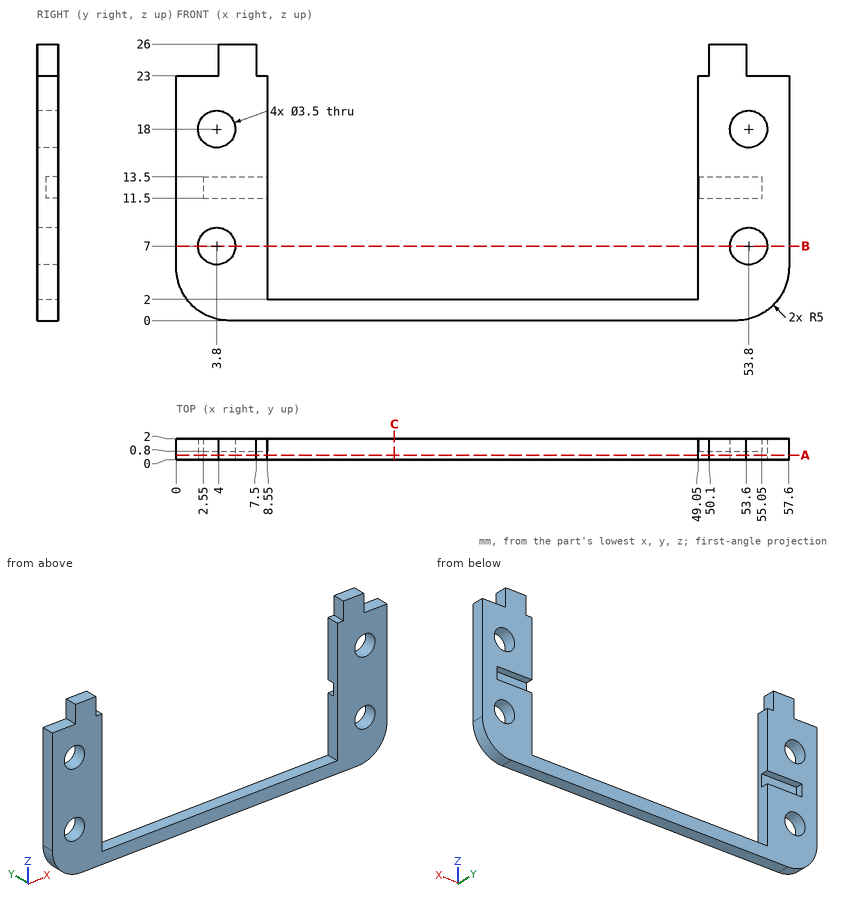
For this review, use the dimensioned drawing (mm, ordinates from the lowest corner) and the shaded views. Coordinates: 2 decimals unless noted, no trailing zeros. Loops run counter-clockwise (first coordinate to the right, second up) from the corner with the lowest first, then second, coordinate; pieces in that order, holes last. Notation, with made-up numbers: (22, 14.25) -> (79, 14.25) arc R23 cw to (79, 31.25) -> close; hole circle Ø2 at (66, 21.5). An arc over 180 degrees is marked (long way). Return JSON: item names as keys, results as strings. Group by question number.
(1) Consider section A-A, the plane y = 0.45. Give the boundary of the cut face in (x, z), plus the area to 3 significant figures.
(2) To check wall thickness, follow L1, parallel to X at y = 1.2, z = 7; L2, parallel to X at y = 1.25, z = 12; L3, parallel to X at y = 0.65, z = 19.5. State the ranges of each line that lie inside material, in increasing order.
(3) For pin 1 Ø8 at (x, z) = (44.5, 13.5) entering from -Y; pin 2 Ø1.6 at (x, z) = (52.5, 12.5) entering from +Y; pin 3 Ø0.6 at (y, z) = (1, 24) entering from -X, all flat-tipped, find the tip position at first contact; note any pin that passes through.
(4) Consider section B-B, the plane z = 7. Give the boundary of the cut face in (x, y).
(5) Consider section C-C, the plane x = 20.5. Give the boundary of the cut face in (y, z), plus the area to 3 significant figures.
Results below:
{
 "1": {"outline": "(0, 5) arc R5 ccw to (5, 0) -> (52.6, 0) arc R5 ccw to (57.6, 5) -> (57.6, 23) -> (53.6, 23) -> (53.6, 26) -> (50.1, 26) -> (50.1, 23) -> (49.05, 23) -> (49.05, 2) -> (8.55, 2) -> (8.55, 23) -> (7.5, 23) -> (7.5, 26) -> (4, 26) -> (4, 23) -> (0, 23) -> close; hole circle Ø3.5 at (3.8, 7); hole circle Ø3.5 at (3.8, 18); hole circle Ø3.5 at (53.8, 7); hole circle Ø3.5 at (53.8, 18)", "area": "446 mm2"},
 "2": {"L1": "x = 0 to 2.05, 5.55 to 8.55, 49.05 to 52.05, 55.55 to 57.6", "L2": "x = 0 to 2.55, 55.05 to 57.6", "L3": "x = 0 to 2.9, 4.7 to 8.55, 49.05 to 52.9, 54.7 to 57.6"},
 "3": {"pin 1": "passes through", "pin 2": "stops at y = 0.8", "pin 3": "stops at x = 4"},
 "4": {"outline": "(0, 0) -> (2.05, 0) -> (2.05, 2) -> (0, 2) -> close; (5.55, 0) -> (8.55, 0) -> (8.55, 2) -> (5.55, 2) -> close; (49.05, 0) -> (52.05, 0) -> (52.05, 2) -> (49.05, 2) -> close; (55.55, 0) -> (57.6, 0) -> (57.6, 2) -> (55.55, 2) -> close"},
 "5": {"outline": "(0, 0) -> (2, 0) -> (2, 2) -> (0, 2) -> close", "area": "4.00 mm2"}
}
